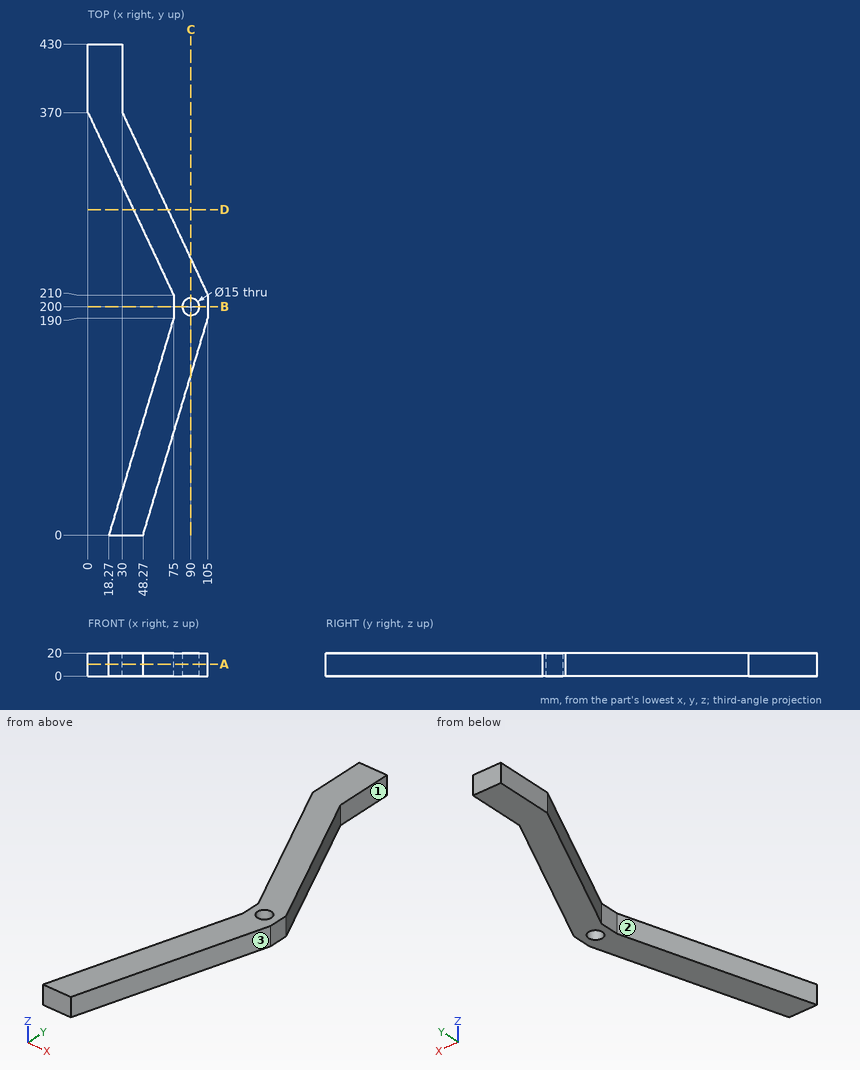
The drawing under review shows one solid part. Ordinate dimensions are in mm from its lowest x, y, z. A direction names the side the tool comes from. Coordinates: 2 decimals unless noted, no trailing zeros. Write each loop counter-clockwise with the first axis right and the second up, starting at its lowest first coordinate (ties: lowest second). Pieces come first, ordered by that corner, then holes. Notation, with made-up numbers: (-11.75, -7) -> (37.25, -7) arc R14 cw to (37.25, -3) -> close; hole circle Ø9 at (27.25, -14). An arc over 180 degrees is marked (long way). Write each question's results on one line, items separated by ' | '. Start each with the question number.
1) Consider section A-A (z = 10.5). Write out the cut boundary in (x, y), plus the area to 3 significant figures.
2) Insertion check: pin 1 (8 mm diameter, centred on y = 168, z = 14, fed in from +X) (1 decimal); pin 2 (12 mm diameter, centred on x = 90, y = 200, fed in from -Z); pin 3 (12 mm diameter, centred on y = 292.5, z = 15, fed in from +X); pin 4 (10 mm diameter, centred on x = 36, z = 8.5, fed in from +Y) (1 decimal). Each pin has a flat end and moves straight along its axis. Give the tip position at first contact, or say it passes through.
3) Consider section B-B (y = 200). Write out the cut boundary in (x, z).
4) Wall thickness on L1, parallel to X at y = 190.5, z = 19; L2, parallel to X at y = 152.5, z = 15.25; L3, parallel to Y at x = 16.5, z = 13.25: over which ranges is each line inside the solid? List them lowest first. Write a range as [from, to].
5) Consider section C-C (x = 90). Write out the cut boundary in (y, z).
6) For the marked faces 1, 2 and 3, list the 3-axis set-ups (+Z, -Z, +X, -X, +Y, -Y) from which the entire face can be reached by the end or side of a thin tool; tool diameter is ignored.
7) Consider section D-D (y = 285). Write out the cut boundary in (x, z).
Geometry says:
1) outline: (0, 370) -> (75, 210) -> (75, 190) -> (18.27, 0) -> (48.27, 0) -> (105, 190) -> (105, 210) -> (30, 370) -> (30, 430) -> (0, 430) -> close; hole circle Ø15 at (90, 200) | area: 12,700 mm^2
2) pin 1: x = 99.6 | pin 2: through | pin 3: x = 69.14 | pin 4: y = 367.9
3) outline: (75, 0) -> (82.5, 0) -> (82.5, 20) -> (75, 20) -> close; (97.5, 0) -> (105, 0) -> (105, 20) -> (97.5, 20) -> close
4) L1: [75, 105] | L2: [63.8, 93.8] | L3: [334.8, 430]
5) outline: (139.76, 0) -> (192.5, 0) -> (192.5, 20) -> (139.76, 20) -> close; (207.5, 0) -> (242, 0) -> (242, 20) -> (207.5, 20) -> close
6) face 1: +Z, -Z, +X, +Y | face 2: +Z, -Z, -X | face 3: +Z, -Z, +X, -Y
7) outline: (39.84, 0) -> (69.84, 0) -> (69.84, 20) -> (39.84, 20) -> close
